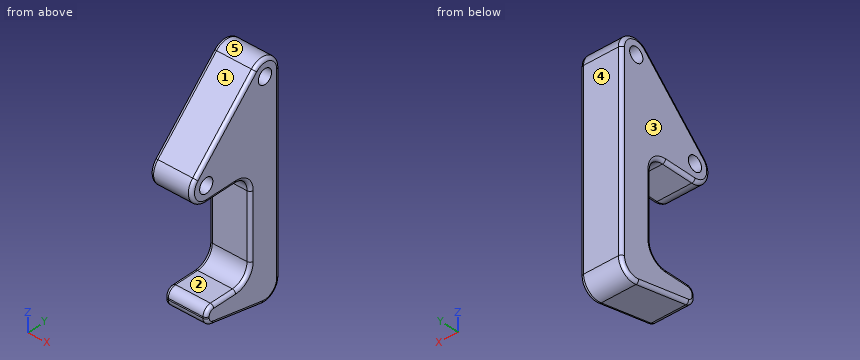
from build123d import *

# Parameters (mm, degrees)
SKETCH1_R           = 2.25
BOSS_EXTRUDE1_DEPTH = 12.7
FILLET1_R           = 5
FILLET2_R           = 2.5
FILLET3_R           = 1


with BuildPart() as part:
    # Sketch1 → Boss-Extrude1 (new body)
    with BuildSketch(Plane(origin=(0, 0, 0), x_dir=(0, 0, -1), z_dir=(1, 0, 0))):
        with BuildLine():
            Line((65, 5), (0, 5))
            ThreePointArc((0, 5), (-4.619397663, 1.913417162), (-3.535533906, -3.535533906))
            Line((-3.535533906, -3.535533906), (16.464466094, -23.535533906))
            ThreePointArc((16.464466094, -23.535533906), (21.913417162, -24.619397663), (25, -20))
            Line((25, -20), (25, -5))
            Line((25, -5), (55, -5))
            Line((55, -5), (55, -20))
            Line((55, -20), (60, -20))
            Line((60, -20), (65, 5))
        make_face()
        Circle(SKETCH1_R, mode=Mode.SUBTRACT)
        with Locations((20, -20)):
            Circle(SKETCH1_R, mode=Mode.SUBTRACT)
    extrude(amount=BOSS_EXTRUDE1_DEPTH)

    # Fillet1
    fillet1_edges = [part.edges().sort_by_distance(p)[0] for p in [
        (6.35, 5, -65),
        (6.35, -5, -55),
        (6.35, -5, -25),
    ]]
    fillet(fillet1_edges, radius=FILLET1_R)

    # Fillet2
    fillet2_edges = [part.edges().sort_by_distance(p)[0] for p in [
        (6.35, -20, -60),
        (6.35, -20, -55),
    ]]
    fillet(fillet2_edges, radius=FILLET2_R)

    # Fillet3
    fillet3_edges = [part.edges().sort_by_distance(p)[0] for p in [
        (12.7, 1.913417162, 4.619397663),
        (0, 5, -29.450490243),
        (0, -24.619397663, -21.913417162),
        (12.7, -13.535533906, -6.464466094),
        (0, -13.535533906, -6.464466094),
        (0, 1.913417162, 4.619397663),
        (12.7, -24.619397663, -21.913417162),
        (0, -5, -40),
        (12.7, -5, -40),
        (0, -15, -25),
        (0, 3.169944528, -62.767691193),
        (12.7, -15, -25),
        (12.7, 3.169944528, -62.767691193),
        (0, -6.464466094, -53.535533906),
        (12.7, -6.464466094, -53.535533906),
        (0, -6.464466094, -26.464466094),
        (12.7, -6.464466094, -26.464466094),
        (12.7, 5, -29.450490243),
        (0, -9.485435507, -62.102912899),
        (12.7, -9.485435507, -62.102912899),
        (0, -20, -57.725245122),
        (0, -13.75, -55),
        (0, -19.267766953, -55.732233047),
        (0, -19.433355353, -59.535462507),
        (12.7, -20, -57.725245122),
        (12.7, -13.75, -55),
        (12.7, -19.267766953, -55.732233047),
        (12.7, -19.433355353, -59.535462507),
    ]]
    fillet(fillet3_edges, radius=FILLET3_R)


solid = part.part
Here's how the part is built. I have some questions about the finished solid (model axes, mm). Face numbers are marked on the shaded views. A direction names the side the tool comes from. Round coordinates to 2 decimals unless told otherwise and drop trailing zeros. Loops run counter-clockwise (first coordinate to the right, second up) from the corner with the lowest first, then second, coordinate; pieces in that order, holes last. Notation, with made-up numbers: (58.5, 64.25) - (88.5, 64.25) arc R28 cw to (88.5, 102.25) - close; hole circle Ø7 at (33, -8). An arc over 180 degrees is marked (long way). One line per question, with ' | ' between items. Start each with the question number.
Q1. Please list where these lines run through material, in increasing order: line 1 (Z direction, x = 2, y = -18.5); line 2 (Y direction, x = 3.25, z = -20); line 3 (Z direction, x = 5.25, y = -18). Write a range as [from, to].
Q2. I want a section at A-A (x = 8). Write out the boundary of the cut face in (y, z).
Q3. We'd pull the mould along Y, two halves only. Please class the marked faces 3, 4 and 5: +Y half, -Y half, draft (parallel to the pull), parting line (faces both ways), or undercut.
Q4. For the marked faces 1 and 2, which set-ups out of +Z, -Z, +X, -X, +Y, -Y let a thin tool reach every point of the face, with its end or its side?
Q5. I want a section at B-B (z = -31). Write out the boundary of the cut face in (x, y).
Q6. Will these pins go through, and if not, where does the flat tip stop? pin 1 (4 mm diameter, centred on x = 5.5, y = -14, fed in from +Z); pin 2 (1 mm diameter, centred on x = 1.5, y = -1, fed in from +Z); pin 3 (3 mm diameter, centred on x = 8.5, z = -44, fed in from -Y).
Response values:
1) line 1: z = [-60.24, -55.21], [-25, -21.68], [-18.32, -11.43] | line 2: y = [-25, -22.25], [-17.75, 5] | line 3: z = [-60.4, -55.05], [-25, -21.03], [-18.97, -10.93]
2) outline: (-23.54, -16.46) arc R5 ccw to (-20, -25) - (-10, -25) arc R5 cw to (-5, -30) - (-5, -50) arc R5 cw to (-10, -55) - (-17.5, -55) arc R2.5 ccw to (-20, -57.5) - (-20, -57.95) arc R2.5 ccw to (-17.99, -60.4) - (-0.98, -63.8) arc R5 ccw to (5, -58.9) - (5, 0) arc R5 ccw to (-3.54, 3.54) - close; hole circle Ø4.5 at (-20, -20); hole circle Ø4.5 at (0, 0)
3) face 3: draft | face 4: +Y half | face 5: parting line
4) face 1: +Z, +X, -X, -Y | face 2: +X, -X, -Y
5) outline: (0, -4) arc R1 ccw to (1, -5) - (11.7, -5) arc R1 ccw to (12.7, -4) - (12.7, 4) arc R1 ccw to (11.7, 5) - (1, 5) arc R1 ccw to (0, 4) - close
6) pin 1: stops at z = -4.93 | pin 2: stops at z = 4.97 | pin 3: stops at y = -5
